from build123d import *

# Parameters (mm, degrees)
F0_W     = 80
F0_H     = 60
F1_DEPTH = 15
F3_D     = 5
F4_R     = 5


with BuildPart() as f1:
    # F0 (on Front) → F1 (new body)
    with BuildSketch(Plane.XZ):
        Rectangle(F0_W, F0_H)
    extrude(amount=F1_DEPTH)

    # F3 (through all)
    with Locations(Plane.XZ.offset(15)):
        with Locations((-30, 20), (30, 20)):
            Hole(F3_D / 2)

    # F4
    f4_edges = [f1.edges().sort_by_distance(p)[0] for p in [
        (40, -7.5, 30),
        (-40, -7.5, 30),
        (-40, -7.5, -30),
        (40, -7.5, -30),
    ]]
    fillet(f4_edges, radius=F4_R)


solid = f1.part
Here's how the part is built. I have some questions about the finished solid (model axes, mm). Coordinates: 2 decimals unless noted, no trailing zeros. Write each loop counter-clockwise with the first axis right and the second up, starting at its lowest first coordinate (ties: lowest second). Pieces come first, ordered by that corner, then holes.
Item 1: If we mould it in two halves opening along Z, with no side actions, what happens to faces 1 (the cylindrical face through (-39, -8, 28)), 2 (the cylindrical face through (-29.67, -7.39, 22.48)), 3 (the flat face through (-40, -7, 0)), 4 (the cylindrical face through (30.33, -7.39, 22.48))? For each: +Z half, -Z half, draft (parallel to the pull), parting line (faces both ways), or undercut.
Item 2: Will this pin go through, and if not, where does the flat tip stop? pin 1 (5 mm diameter, centred on x = 23.5, z = -20, fed in from +Y).
Item 3: I want a section at A-A on x = 30. Write out the boundary of the cut face in (y, z), and give its area (3 significant figures).
Item 4: If I drill on line 1 (Z direction, x = -30, y = -6); line 2 (X direction, y = -2.75, z = 18.5); line 3 (Z direction, x = 29.5, y = -10.5), over which ranges is the centre line in solid material (lowest first)?
Item 5: I want a section at B-B on z = 20. Write out the boundary of the cut face in (x, y).
Findings below:
1. face 1: +Z half
1. face 2: undercut
1. face 3: draft
1. face 4: undercut
2. pin 1: stops at y = 0
3. outline: (-15, -30) - (0, -30) - (0, 17.5) - (-15, 17.5) - close; (-15, 22.5) - (0, 22.5) - (0, 30) - (-15, 30) - close
3. area: 825 mm2
4. line 1: z = -30 to 17.5, 22.5 to 30
4. line 2: x = -40 to -32, -28 to 28, 32 to 40
4. line 3: z = -30 to 17.55, 22.45 to 30
5. outline: (-40, -15) - (-32.5, -15) - (-32.5, 0) - (-40, 0) - close; (-27.5, -15) - (27.5, -15) - (27.5, 0) - (-27.5, 0) - close; (32.5, -15) - (40, -15) - (40, 0) - (32.5, 0) - close
